Here's how the part is built. I have some questions about the finished solid (model axes, mm). A direction names the side the tool comes from. Round coordinates to 2 decimals unless told otherwise and drop trailing zeros. Order: outer loops, then holes, each group sorted by start corner. A loop starts at its lowest first (then second) coordinate and runs counter-clockwise, first axis right, second up. Notation, with made-up numbers: M 43.5,-13 L 84.5,-13 A30 cw 84.5,25 Z; hole C 30,-3 d10. An arc over 180 degrees is marked long. Write each question's results on one line, items separated by ' | '. Start each with the question number.
```python
from build123d import *

# Parameters (mm, degrees)
SKETCH1_R           = 7.9502
SKETCH1_R_2         = 1.524
SKETCH1_R_3         = 2.9845
SKETCH1_R_4         = 7.250000001
BOSS_EXTRUDE1_DEPTH = 12.7
SKETCH1_3_R         = 7.9502
SKETCH1_3_R_2       = 7.250000001
CUT_EXTRUDE1_DEPTH  = 4.699
CUT_EXTRUDE2_START  = 6.35
SKETCH1_4_R         = 2.9845
CUT_EXTRUDE2_DEPTH  = 6.35


with BuildPart() as part:
    # Sketch1 → Boss-Extrude1 (new body)
    # profile 1 of 3: a face of its own
    with BuildSketch(Plane.XY):
        with BuildLine():
            Line((125.367960427, 117.540284058), (125.367960427, 83.715284058))
            Line((125.367960427, 83.715284058), (153.367960426, 83.715284058))
            Line((153.367960426, 83.715284058), (153.367960426, 117.540284058))
            ThreePointArc((153.367960426, 117.540284058), (152.438024457, 119.785348088), (150.192960426, 120.715284058))
            Line((150.192960426, 120.715284058), (128.542960427, 120.715284058))
            ThreePointArc((128.542960427, 120.715284058), (126.297896397, 119.785348088), (125.367960427, 117.540284058))
        make_face()
        with Locations((139.367960428, 109.715284059)):
            Circle(SKETCH1_R, mode=Mode.SUBTRACT)
        with Locations((150.162960428, 109.715284059)):
            Circle(SKETCH1_R_2, mode=Mode.SUBTRACT)
    # profile 2 of 3: a face of its own
    with BuildSketch(Plane.XY):
        with BuildLine():
            ThreePointArc((125.367960427, 67.360204058), (126.297896397, 65.115140027), (128.542960427, 64.185204058))
            Line((128.542960427, 64.185204058), (150.192960426, 64.185204058))
            ThreePointArc((150.192960426, 64.185204058), (152.438024457, 65.115140027), (153.367960426, 67.360204058))
            Line((153.367960426, 67.360204058), (153.367960426, 83.715284058))
            Line((153.367960426, 83.715284058), (125.367960427, 83.715284058))
            Line((125.367960427, 83.715284058), (125.367960427, 67.360204058))
        make_face()
        with Locations((131.367960426, 73.715284058)):
            Circle(SKETCH1_R_3, mode=Mode.SUBTRACT)
        with Locations((147.367960427, 73.715284058)):
            Circle(SKETCH1_R_3, mode=Mode.SUBTRACT)
    # profile 3 of 3: a face of its own
    with BuildSketch(Plane.XY):
        with Locations((139.367960428, 109.715284059)):
            Circle(SKETCH1_R)
        with Locations((139.367960428, 109.715284059)):
            Circle(SKETCH1_R_4, mode=Mode.SUBTRACT)
    extrude(amount=BOSS_EXTRUDE1_DEPTH)

    # Sketch1<3> → Cut-Extrude1 (cut)
    with BuildSketch(Plane.XY):
        with Locations((139.367960428, 109.715284059)):
            Circle(SKETCH1_3_R)
        with Locations((139.367960428, 109.715284059)):
            Circle(SKETCH1_3_R_2, mode=Mode.SUBTRACT)
    extrude(amount=CUT_EXTRUDE1_DEPTH, mode=Mode.SUBTRACT)

    # Sketch1<4> → Cut-Extrude2 (cut)
    with BuildSketch(Plane.XY.offset(CUT_EXTRUDE2_START)):
        with BuildLine():
            ThreePointArc((125.367960427, 67.360204058), (126.297896397, 65.115140027), (128.542960427, 64.185204058))
            Line((128.542960427, 64.185204058), (150.192960426, 64.185204058))
            ThreePointArc((150.192960426, 64.185204058), (152.438024457, 65.115140027), (153.367960426, 67.360204058))
            Line((153.367960426, 67.360204058), (153.367960426, 83.715284058))
            Line((153.367960426, 83.715284058), (125.367960427, 83.715284058))
            Line((125.367960427, 83.715284058), (125.367960427, 67.360204058))
        make_face()
        with Locations((131.367960426, 73.715284058)):
            Circle(SKETCH1_4_R, mode=Mode.SUBTRACT)
        with Locations((147.367960427, 73.715284058)):
            Circle(SKETCH1_4_R, mode=Mode.SUBTRACT)
    extrude(amount=CUT_EXTRUDE2_DEPTH, mode=Mode.SUBTRACT)


solid = part.part
```
(1) If we mould it in two halves opening along X, with no side actions, what happens to faces 4 (the flat face through (153.368, 98, 6)), 5 (the flat face through (139, 64.185, 3)), 6 (the cylindrical face through (150.215, 74.612, 3.131)), 7 (the flat face through (143, 103, 4.699))? For each: pulls with the +X half, pulls with the -X half, needs draft (parallel to the pull), parting line crosses it, or undercut.
(2) I want a section at B-B on y = 72. Write out the boundary of the cut face in (x, z), and give its area (3 significant figures).
(3) I want a section at D-D on y = 105. Write out the boundary of the cut face in (x, z).
(4) I want a section at C-C on z = 2.5. Give the number of separate pieces and of enclosed holes in the cut face, and give its area (3 significant figures).
(5) Please list where these lines run through material, in increasing order: line 1 (X direction, y = 111, z = 6.25); line 2 (Y direction, x = 132.75, z = 5); line 3 (Z direction, x = 128, y = 79.5).
(6) On a 3-axis mill with a long thin cutter (end or side, diameter ignored), from which of +Z, -Z, +X, -X, +Y, -Y can I reach the whole of each face in a straight line? I mean faces 1 (the cylindrical face through (126.32, 119.81, 6.26)), 2 (the flat face through (140, 83.715, 9)), 3 (the cylindrical face through (131.425, 110.065, 2.317)). Say none if no direction works.
(7) I want a section at A-A on x = 137.5. Write out the boundary of the cut face in (y, z), and give its area (3 significant figures).
(8) I'm going to push flat-ended pins straight in: pin 1 Ø9.5 at (x, y) = (147.37, 73.72) entering from +Z; pin 2 Ø5 at (x, z) = (141, 10.5) entering from -Y. Where does each tip first touch, or does it pass through?
Solutions:
1) face 4: pulls with the +X half | face 5: needs draft | face 6: undercut | face 7: undercut
2) outline: M 125.37,0 L 128.93,0 L 128.93,6.35 L 125.37,6.35 Z; M 133.81,0 L 144.93,0 L 144.93,6.35 L 133.81,6.35 Z; M 149.81,0 L 153.37,0 L 153.37,6.35 L 149.81,6.35 Z | area: 116 mm^2
3) outline: M 125.37,0 L 132.97,0 L 132.97,4.7 L 133.86,4.7 L 133.86,12.7 L 125.37,12.7 Z; M 144.88,4.7 L 145.77,4.7 L 145.77,0 L 153.37,0 L 153.37,12.7 L 144.88,12.7 Z
4) separate pieces: 1 | enclosed holes: 4 | area: 1,310 mm^2
5) line 1: 125.37 to 132.23, 146.5 to 149.34, 150.98 to 153.37 | line 2: 64.19 to 71.07, 76.36 to 106.75, 112.68 to 120.72 | line 3: 0 to 6.35
6) face 1: +Z, -Z, -X, +Y | face 2: +Z, +X, -X, -Y | face 3: -Z
7) outline: M 64.19,0 L 101.99,0 L 101.99,4.7 L 102.71,4.7 L 102.71,12.7 L 83.72,12.7 L 83.72,6.35 L 64.19,6.35 Z; M 116.72,4.7 L 117.44,4.7 L 117.44,0 L 120.72,0 L 120.72,12.7 L 116.72,12.7 Z | area: 409 mm^2
8) pin 1: z = 6.35 | pin 2: y = 83.72
